Here's the drawing with two shaded views (mm, measured from the low corner). I have some questions. A direction names the side the tool comes from. Round coordinates to 2 decimals unless told otherwise and drop trailing zeros. Order: outer loops, then holes, each group sorted by start corner. A loop starts at its lowest first (then second) coordinate and runs counter-clockwise, first axis right, second up.
Q1. We'd pull the mould along Y, two halves only. Please class the marked faces 4, 5 and 6: pulls with the +Y half, pulls with the -Y half, needs draft (parallel to the pull), parting line crosses it, or undercut.
Q2. If we section it at C-C (x = 7.25): Please give me the cut outline in (y, z), plus the area to 3 significant figures.
Q3. For the marked faces 1, 2 and 3, which set-ups out of +Z, -Z, +X, -X, +Y, -Y let a thin tool reach every point of the face, with its end or its side?
Q4. If we section it at D-D (y = 13): Please give me the cut outline in (x, z).
Q5. Will these pins go through, and if not, where does the flat tip stop? P1, Ø4, axis at y = 40, z = 6.5, coming from the -X side (1 decimal); P2, Ø2, axis at x = 17, z = 14, coming from the +Y side; P3, Ø1.5, axis at y = 39, z = 5.5, coming from the +X side.
Q6. If I drill on line 1 (Y direction, x = 11.5, z = 15) (1 decimal); line 2 (X direction, y = 6, z = 3) (1 decimal); line 3 (Y direction, x = 2.5, z = 10.75) (1 decimal), over which ranges is the centre line in solid material (lowest first)?
Q7. If we section it at A-A (y = 27.5): Please give me the cut outline in (x, z) (1 decimal).
Q8. If we section it at B-B (z = 8.5): Please give me the cut outline in (x, y) (1 decimal).
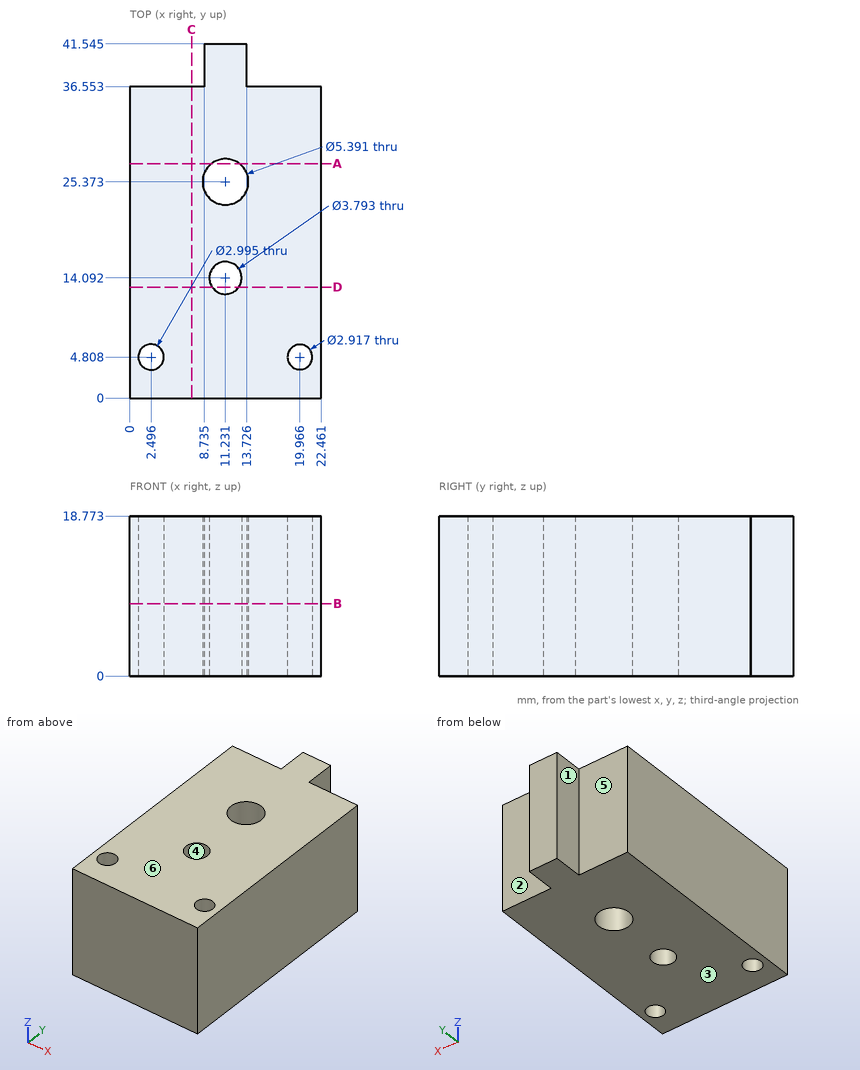
Solution:
1. face 4: undercut
1. face 5: pulls with the +Y half
1. face 6: needs draft
2. outline: (0, 0) - (36.55, 0) - (36.55, 18.77) - (0, 18.77) - close
2. area: 686 mm2
3. face 1: +Z, -Z, -X, +Y
3. face 2: +Z, -Z, +X, +Y
3. face 3: -Z, +X, -X, +Y, -Y
4. outline: (0, 0) - (9.68, 0) - (9.68, 18.77) - (0, 18.77) - close; (12.78, 0) - (22.46, 0) - (22.46, 18.77) - (12.78, 18.77) - close
5. P1: stops at x = 8.7
5. P2: stops at y = 36.55
5. P3: stops at x = 13.73
6. line 1: y = 0 to 12.2, 16 to 22.7, 28.1 to 41.5
6. line 2: x = 0 to 1.6, 3.4 to 19.1, 20.8 to 22.5
6. line 3: y = 0 to 3.3, 6.3 to 36.6
7. outline: (0, 0) - (9.6, 0) - (9.6, 18.8) - (0, 18.8) - close; (12.9, 0) - (22.5, 0) - (22.5, 18.8) - (12.9, 18.8) - close
8. outline: (0, 0) - (22.5, 0) - (22.5, 36.6) - (13.7, 36.6) - (13.7, 41.5) - (8.7, 41.5) - (8.7, 36.6) - (0, 36.6) - close; hole circle Ø3 at (2.5, 4.8); hole circle Ø5.4 at (11.2, 25.4); hole circle Ø3.8 at (11.2, 14.1); hole circle Ø2.9 at (20, 4.8)
